from build123d import *

# Parameters (mm, degrees)
SKETCH16_W          = 44
SKETCH16_H          = 35
SKETCH16_R          = 1.25
BOSS_EXTRUDE1_DEPTH = 8
SKETCH1_R           = 4
CUT_EXTRUDE3_DEPTH  = 9


with BuildPart() as part:
    # Sketch16 → Boss-Extrude1 (new body)
    with BuildSketch(Plane(origin=(0, 0, 0), x_dir=(-1, 0, 0), z_dir=(0, 1, 0))):
        Rectangle(SKETCH16_W, SKETCH16_H)
        with Locations((-19, 14.5)):
            Circle(SKETCH16_R, mode=Mode.SUBTRACT)
        with Locations((19, 14.5)):
            Circle(SKETCH16_R, mode=Mode.SUBTRACT)
        with Locations((19, -14.5)):
            Circle(SKETCH16_R, mode=Mode.SUBTRACT)
        with Locations((-19, -14.5)):
            Circle(SKETCH16_R, mode=Mode.SUBTRACT)
    extrude(amount=BOSS_EXTRUDE1_DEPTH)

    # Sketch1 → Cut-Extrude3 (cut, through all)
    with BuildSketch(Plane(origin=(0, 0, 0), x_dir=(1, 0, 0), z_dir=(0, 1, 0))):
        Circle(SKETCH1_R)
    extrude(amount=CUT_EXTRUDE3_DEPTH, mode=Mode.SUBTRACT)


solid = part.part
Could you check a few things on this model? Use its own coordinates, in mm. Coordinates: 2 decimals unless noted, no trailing zeros. Order: outer loops, then holes, each group sorted by start corner. A loop starts at its lowest first (then second) coordinate and runs counter-clockwise, first axis right, second up.
Q1. Will this pin go through, and if not, where does the flat tip stop? pin 1 (4 mm diameter, centred on x = 19, z = 14.5, fed in from -Y).
Q2. Suppose I cut it at A-A on z = 0. Please give me the cut outline in (x, y), and give its area (3 significant figures).
Q3. Suppose I cut it at B-B on z = -14.5. Please give me the cut outline in (x, y), and give its area (3 significant figures).
Q4. Please list where these lines run through material, in increasing order: L1, parallel to Z at x = -19, y = 4; L2, parallel to Z at x = 0, y = 2; L3, parallel to X at y = 1, z = -1.5.
Q5. Thinking about a two-plate mould opening in Z: for faces 1 (the cylindrical face through (18.328, 3.944, 15.554)), 2 (the flat face through (5, 0, 0)), 3 (the flat face through (0, 4, 17.5)), 4 (the flat face through (0, 4, -17.5)), which applies, released by +Z, released by -Z, zero draft, split by the parting line, or undercut?
Q6. Suppose I cut it at C-C on x = 0. Please give me the cut outline in (y, z), and give its area (3 significant figures).
Q7. Suppose I cut it at D-D on x = -19. Please give me the cut outline in (y, z), and give its area (3 significant figures).
Answer:
1. pin 1: stops at y = 0
2. outline: (-22, 0) - (-4, 0) - (-4, 8) - (-22, 8) - close; (4, 0) - (22, 0) - (22, 8) - (4, 8) - close
2. area: 288 mm2
3. outline: (-22, 0) - (-20.25, 0) - (-20.25, 8) - (-22, 8) - close; (-17.75, 0) - (17.75, 0) - (17.75, 8) - (-17.75, 8) - close; (20.25, 0) - (22, 0) - (22, 8) - (20.25, 8) - close
3. area: 312 mm2
4. L1: z = -17.5 to -15.75, -13.25 to 13.25, 15.75 to 17.5
4. L2: z = -17.5 to -4, 4 to 17.5
4. L3: x = -22 to -3.71, 3.71 to 22
5. face 1: undercut
5. face 2: zero draft
5. face 3: released by +Z
5. face 4: released by -Z
6. outline: (0, -17.5) - (8, -17.5) - (8, -4) - (0, -4) - close; (0, 4) - (8, 4) - (8, 17.5) - (0, 17.5) - close
6. area: 216 mm2
7. outline: (0, -17.5) - (8, -17.5) - (8, -15.75) - (0, -15.75) - close; (0, -13.25) - (8, -13.25) - (8, 13.25) - (0, 13.25) - close; (0, 15.75) - (8, 15.75) - (8, 17.5) - (0, 17.5) - close
7. area: 240 mm2
